```python
from build123d import *

# Parameters (mm, degrees)
SKETCH_1_W          = 19
SKETCH_1_H          = 19
SKETCH_1_W_2        = 13
SKETCH_1_H_2        = 13
EXTRUDE_1_DEPTH     = 85.9
SKETCH_2_R          = 1.65
CUT_EXTRUDE_1_DEPTH = 30
SKETCH_3_W          = 116.915177823
SKETCH_3_H          = 46.219516436
CUT_EXTRUDE_2_DEPTH = 3
SKETCH_4_W          = 5
SKETCH_4_H          = 13
EXTRUDE_1_2_DEPTH   = 10
SKETCH_5_W          = 29.9
SKETCH_5_H          = 5
EXTRUDE_2_DEPTH     = 10
SKETCH_6_W          = 39.9
SKETCH_6_H          = 13
EXTRUDE_3_DEPTH     = 10
SKETCH_8_W          = 39.9
SKETCH_8_H          = 5
CUT_EXTRUDE_3_DEPTH = 3
CHAMFER_1_SIZE      = 3
CHAMFER_2_SIZE      = 4


with BuildPart() as part:
    # 草图1 → Extrude 1 (new body)
    with BuildSketch(Plane.XY):
        with Locations((6.5, 6.5)):
            Rectangle(SKETCH_1_W, SKETCH_1_H)
        with Locations((6.5, 6.5)):
            Rectangle(SKETCH_1_W_2, SKETCH_1_H_2, mode=Mode.SUBTRACT)
    extrude(amount=EXTRUDE_1_DEPTH)

    # 草图2 → 切除-拉伸1 (cut)
    with BuildSketch(Plane.ZY.offset(3)):
        with Locations((10, 6.5)):
            Circle(SKETCH_2_R)
        with Locations((75.9, 6.5)):
            Circle(SKETCH_2_R)
    extrude(amount=-CUT_EXTRUDE_1_DEPTH, mode=Mode.SUBTRACT)

    # 草图3 → 切除-拉伸2 (cut)
    with BuildSketch(Plane.ZY.offset(3)):
        with Locations((53.162237228, 0.202739406)):
            Rectangle(SKETCH_3_W, SKETCH_3_H)
    extrude(amount=-CUT_EXTRUDE_2_DEPTH, mode=Mode.SUBTRACT)

    # 草图4 → Extrude 1 2 (add)
    with BuildSketch(Plane.ZY.offset(-13)):
        with Locations((25.5, 6.5)):
            Rectangle(SKETCH_4_W, SKETCH_4_H)
        with Locations((60.4, 6.5)):
            Rectangle(SKETCH_4_W, SKETCH_4_H)
    extrude(amount=EXTRUDE_1_2_DEPTH)

    # 草图5 → 凸台-拉伸2 (add)
    with BuildSketch(Plane.ZY.offset(-13)):
        with Locations((42.95, 6.5)):
            Rectangle(SKETCH_5_W, SKETCH_5_H)
    extrude(amount=EXTRUDE_2_DEPTH)

    # 草图6 → 凸台-拉伸3 (add)
    with BuildSketch(Plane.ZY.offset(-13)):
        with Locations((42.95, 6.5)):
            Rectangle(SKETCH_6_W, SKETCH_6_H)
    extrude(amount=EXTRUDE_3_DEPTH)

    # 草图8 → 切除-拉伸3 (cut)
    with BuildSketch(Plane.ZY.offset(-3)):
        with Locations((42.95, 6.5)):
            Rectangle(SKETCH_8_W, SKETCH_8_H)
    extrude(amount=-CUT_EXTRUDE_3_DEPTH, mode=Mode.SUBTRACT)

    # 倒角1
    chamfer_1_edges = [part.edges().sort_by_distance(p)[0] for p in [
        (6, 6.5, 23),
        (6, 6.5, 62.9),
    ]]
    chamfer(chamfer_1_edges, length=CHAMFER_1_SIZE)

    # 倒角2
    chamfer_2_edges = [part.edges().sort_by_distance(p)[0] for p in [
        (13, 6.5, 23),
        (13, 6.5, 62.9),
    ]]
    chamfer(chamfer_2_edges, length=CHAMFER_2_SIZE - 0.0001)  # a hair under: the kernel refuses the full size


solid = part.part
```
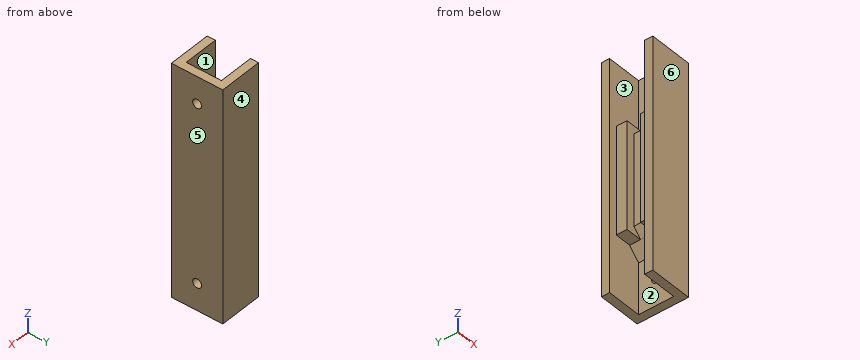
Input: part model. Units: mm. Frame: model coordinates. Face numbers are marked on the shaded views. A direction names the side the tool comes from. Coordinates: 2 decimals unless noted, no trailing zeros. Write each loop counter-clockwise with the first axis right and the second up, starting at its lowest first coordinate (ties: lowest second). Pieces come first, ordered by that corner, then holes. Notation, with made-up numbers: (12.5, 37.5) -> (38.5, 37.5) arc R14 ccw to (38.5, 57.5) -> close; hole circle Ø3 at (88.5, 0.25). An arc over 180 degrees is marked (long way). Write each question's results on one line, items separated by ' | '.
Item 1: Mould query, pull axis Y, two halves, no side actions, for the marked faces 3, 4, 5 and 6. Classes: +Y half, -Y half, draft (parallel to the pull), parting line (faces both ways), or undercut.
Conclusion:
face 3: undercut | face 4: +Y half | face 5: draft | face 6: -Y half
Item 2: Section query C-C on x = 6.75. Return loops of the section in (y, z).
Conclusion:
outline: (-3, 0) -> (0, 0) -> (0, 23) -> (4, 23) -> (4, 25.25) -> (9, 25.25) -> (9, 23) -> (13, 23) -> (13, 0) -> (16, 0) -> (16, 85.9) -> (13, 85.9) -> (13, 62.9) -> (9, 62.9) -> (9, 60.65) -> (4, 60.65) -> (4, 62.9) -> (0, 62.9) -> (0, 85.9) -> (-3, 85.9) -> close
Item 3: Section query D-D on z = 40. Return loops of the section in (x, y), plus the area to 3 significant figures.
Conclusion:
outline: (0, -3) -> (16, -3) -> (16, 16) -> (0, 16) -> (0, 13) -> (3, 13) -> (3, 9) -> (6, 9) -> (6, 4) -> (3, 4) -> (3, 0) -> (0, 0) -> close | area: 250 mm^2
Item 4: Pin query (flat end, axial travel): pin 1 Ø4.5 at (y, z) = (10.5, 38) entering from -X; pin 2 Ø1.8 at (x, y) = (5.5, 8.5) entering from +Z; pin 3 Ø3 at (y, z) = (6, 25) entering from -X; pin 4 Ø2 at (y, z) = (6.5, 10) entering from +X. Return the tip coordinate at first contact, or that it passes through.
Conclusion:
pin 1: stops at x = 3 | pin 2: stops at z = 62.9 | pin 3: stops at x = 6 | pin 4: passes through
Item 5: Section query A-A on y = 6.5. Count the separate pieces of the cut face and the enclosed holes in it, plus the area to 3 significant figures.
Conclusion:
separate pieces: 3 | enclosed holes: 0 | area: 524 mm^2
Item 6: Material intervals for probe 1 along Y at (x, z) = (14.5, 10); probe 2 along Y at (x, z) = (1.5, 81); probe 3 along Z at (x, y) = (3.5, 0.25), sorted ascending.
Conclusion:
probe 1: y = -3 to 4.85, 8.15 to 16 | probe 2: y = -3 to 0, 13 to 16 | probe 3: z = 23 to 62.9
Item 7: Set-up query: the marked faces 1 and 2. Return all of +Z, -Z, +X, -X, +Y, -Y with unobstructed straight access to the full face (end or side cutting, diameter ignored); none if empty.
Conclusion:
face 1: -X | face 2: -Z, -X
Item 8: Section query B-B on z = 75.9. Return loops of the section in (x, y).
Conclusion:
outline: (0, -3) -> (16, -3) -> (16, 4.85) -> (13, 4.85) -> (13, 0) -> (0, 0) -> close; (0, 13) -> (13, 13) -> (13, 8.15) -> (16, 8.15) -> (16, 16) -> (0, 16) -> close
